Build history of the part. All positions in model axes, mm. Face numbers are marked on the shaded views. A direction names the side the tool comes from. Give positions to 0.01 mm unless a question says otherwise; leave off trailing zeros. Order: outer loops, then holes, each group sorted by start corner. A loop starts at its lowest first (then second) coordinate and runs counter-clockwise, first axis right, second up. Notation, with made-up numbers: (-18.75, 58) - (20.25, 58) arc R18 ccw to (20.25, 71) - close; hole circle Ø5 at (-30, -0.5). An arc over 180 degrees is marked (long way). Answer in a Markdown table with one row per item.
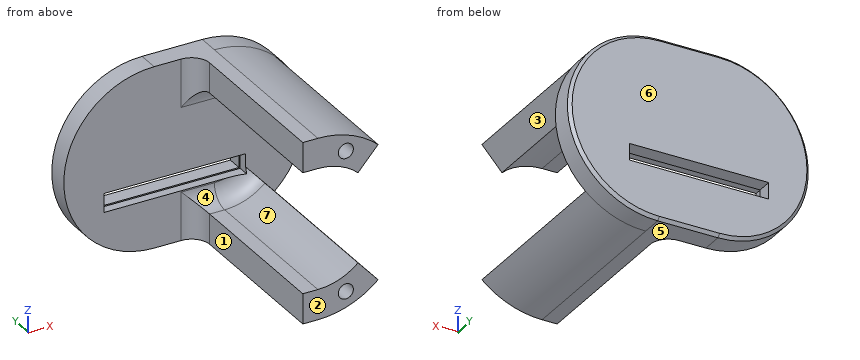
```python
from build123d import *

# Parameters (mm, degrees)
AUFSATZ_LINEAR_AUSTRAGEN1_DEPTH   = 30
AUFSATZ_LINEAR_AUSTRAGEN1_2_DEPTH = 30
AUFSATZ_LINEAR_AUSTRAGEN2_DEPTH   = 4
VERRUNDUNG1_R                     = 3
VERRUNDUNG2_R                     = 3
FASE1_SIZE                        = 0.5
SKIZZE3_R                         = 1.25
SCHNITT_LINEAR_AUSTRAGEN1_DEPTH   = 8
SKIZZE4_W                         = 23.1
SKIZZE4_H                         = 2.74
SCHNITT_LINEAR_AUSTRAGEN2_DEPTH   = 2.5
SCHNITT_LINEAR_AUSTRAGEN3_REACH   = 33.5
SKIZZE5_W                         = 23.5
SKIZZE5_H                         = 3.14


with BuildPart() as part:
    # Skizze1 → Aufsatz-Linear austragen1 (new body)
    with BuildSketch(Plane(origin=(0, 0, 0), x_dir=(1, 0, 0), z_dir=(0, 1, 0))):
        with BuildLine():
            Line((5, 15), (2.5, 15))
            Line((2.5, 15), (2.5, 10))
            Line((2.5, 10), (5, 10))
            ThreePointArc((5, 10), (8.568220898, 9.34172359), (11.666666667, 7.453559925))
            Line((11.666666667, 7.453559925), (15, 11.180339887))
            ThreePointArc((15, 11.180339887), (10.352331347, 14.012585384), (5, 15))
        make_face()
    extrude(amount=-AUFSATZ_LINEAR_AUSTRAGEN1_DEPTH)



with BuildPart() as body_2:
    # Skizze1 → Aufsatz-Linear austragen1 2 (new body)
    with BuildSketch(Plane(origin=(0, 0, 0), x_dir=(1, 0, 0), z_dir=(0, 1, 0))):
        with BuildLine():
            Line((11.666666667, -7.453559925), (15, -11.180339887))
            ThreePointArc((15, -11.180339887), (10.352331347, -14.012585384), (5, -15))
            Line((5, -15), (2.5, -15))
            Line((2.5, -15), (2.5, -10))
            Line((2.5, -10), (5, -10))
            ThreePointArc((5, -10), (8.568220898, -9.34172359), (11.666666667, -7.453559925))
        make_face()
    extrude(amount=-AUFSATZ_LINEAR_AUSTRAGEN1_2_DEPTH)


with BuildPart() as part_1:
    add(part.part)

    add(body_2.part)  # Aufsatz-Linear austragen2 merges body 2
    # Skizze2 → Aufsatz-Linear austragen2 (add)
    with BuildSketch(Plane(origin=(0, 0, 0), x_dir=(1, 0, 0), z_dir=(0, 1, 0))):
        with BuildLine():
            Line((-5, 15), (5, 15))
            ThreePointArc((5, 15), (20, 0), (5, -15))
            Line((5, -15), (-5, -15))
            ThreePointArc((-5, -15), (-20, 0), (-5, 15))
        make_face()
    extrude(amount=AUFSATZ_LINEAR_AUSTRAGEN2_DEPTH)

    # Verrundung1
    verrundung1_edges = [part_1.edges().sort_by_distance(p)[0] for p in [
        (8.568220898, 0, 9.34172359),
        (3.75, 0, 10),
        (8.568220898, 0, -9.34172359),
        (3.75, 0, -10),
    ]]
    fillet(verrundung1_edges, radius=VERRUNDUNG1_R)

    # Verrundung2
    verrundung2_edges = [part_1.edges().sort_by_distance(p)[0] for p in [
        (2.5, 0, 12.5),
        (2.5, 0, -12.5),
    ]]
    fillet(verrundung2_edges, radius=VERRUNDUNG2_R)

    # Fase1
    fase1_edges = [part_1.edges().sort_by_distance(p)[0] for p in [
        (-20, 4, 0),
        (0, 4, 15),
        (20, 4, 0),
        (0, 4, -15),
    ]]
    chamfer(fase1_edges, length=FASE1_SIZE)

    # Skizze3 → Schnitt-Linear austragen1 (cut)
    with BuildSketch(Plane.XZ.offset(30)):
        with Locations((9.644187298, -11.605236936)):
            Circle(SKIZZE3_R)
        with Locations((9.644187298, 11.605236936)):
            Circle(SKIZZE3_R)
    extrude(amount=-SCHNITT_LINEAR_AUSTRAGEN1_DEPTH, mode=Mode.SUBTRACT)

    # Skizze4 → Schnitt-Linear austragen2 (cut)
    with BuildSketch(Plane(origin=(0, 4, 0), x_dir=(1, 0, 0), z_dir=(0, 1, 0))):
        with Locations((-1.602471757, 5.205199937)):
            Rectangle(SKIZZE4_W, SKIZZE4_H)
    extrude(amount=-SCHNITT_LINEAR_AUSTRAGEN2_DEPTH, mode=Mode.SUBTRACT)

    # Skizze5 → Schnitt-Linear austragen3 (cut, up to next)
    with BuildSketch(Plane(origin=(0, 1.5, 0), x_dir=(1, 0, 0), z_dir=(0, 1, 0)), mode=Mode.PRIVATE) as schnitt_linear_austragen3_sk1:
        with Locations((-1.602471757, 5.205199937)):
            Rectangle(SKIZZE5_W, SKIZZE5_H)
    schnitt_linear_austragen3_tool1 = extrude(schnitt_linear_austragen3_sk1.sketch, amount=-SCHNITT_LINEAR_AUSTRAGEN3_REACH, mode=Mode.PRIVATE) & part_1.part
    add(schnitt_linear_austragen3_tool1.solids().sort_by_distance((-1.602472, 1.5, -5.2052))[0], mode=Mode.SUBTRACT)


solid = part_1.part
```
1. Cut at C-C on y = -2.5. Write the cut outline in (x, z).
Check result:
| item | result |
|---|---|
| outline | (2.46, -15) - (5, -15) arc R15 ccw to (15, -11.18) - (11.64, -7.42) arc R9.96 cw to (5, -9.96) - (2.46, -9.96) - close; (2.46, 9.96) - (5, 9.96) arc R9.96 cw to (11.64, 7.42) - (15, 11.18) arc R15 ccw to (5, 15) - (2.46, 15) - close |
2. Which spindle directions (+Z, -Z, +X, -X, +Y, -Y) get a long thin tool onto all of the face, cutting with end or side? Do the marked faces 1, 2, 3 and 4. Say none if no direction does.
Check result:
| item | result |
|---|---|
| face 1 | +Z, -Z, -X, -Y |
| face 2 | +Z, -Z, +X, -X, -Y |
| face 3 | +X, -Y |
| face 4 | -X, -Y |
3. Cut at D-D on x = -2.5. Write the cut outline in (y, z), and give its area (3 significant figures).
Check result:
| item | result |
|---|---|
| outline | (0, -15) - (3.5, -15) - (4, -14.5) - (4, -6.58) - (1.5, -6.58) - (1.5, -6.78) - (0, -6.78) - close; (0, -3.64) - (1.5, -3.64) - (1.5, -3.84) - (4, -3.84) - (4, 14.5) - (3.5, 15) - (0, 15) - close |
| area | 108 mm² |
4. Drop flat-ended pins along their axis: P1, Ø1.5, axis at x = -1.5, y = -2.5, coming from the +Z side; P2, Ø3.5, axis at x = -2.5, z = -4.5, coming from the -Y side; P3, Ø5.5, axis at y = -14.5, z = -13, coming from the -X side; P4, Ø1.2, axis at y = 0.5, z = -5.5, coming from the +X side. Give the stop position or say it passes through.
Check result:
| item | result |
|---|---|
| P1 | passes through |
| P2 | stops at y = 0 |
| P3 | stops at x = 2.5 |
| P4 | stops at x = 19.18 |
5. Cut at A-A on x = 4.5. Write the cut outline in (y, z).
Check result:
| item | result |
|---|---|
| outline | (-30, -15) - (3.5, -15) - (4, -14.5) - (4, -6.58) - (1.5, -6.58) - (1.5, -6.78) - (0, -6.78) - (0, -7) arc R3 cw to (-3, -10) - (-30, -10) - close; (-30, 10) - (-3, 10) arc R3 cw to (0, 7) - (0, -3.64) - (1.5, -3.64) - (1.5, -3.84) - (4, -3.84) - (4, 14.5) - (3.5, 15) - (-30, 15) - close |
6. Two-plate mould, pull along Z, no slides. Class the marked faces 5, 6 and 7: +Z half, -Z half, draft (parallel to the pull), parting line (faces both ways), or undercut.
Check result:
| item | result |
|---|---|
| face 5 | -Z half |
| face 6 | draft |
| face 7 | undercut |
7. Cut at B-B on z = 0. Write the cut outline in (x, y), and give its area (3 significant figures).
Check result:
| item | result |
|---|---|
| outline | (-20, 0) - (20, 0) - (20, 3.5) - (19.5, 4) - (-19.5, 4) - (-20, 3.5) - close |
| area | 160 mm² |
8. Probe line 1 (Z direction, x = 5, y = -6.5); line 2 (Z direction, x = 9, y = -23); line 3 (Y direction, x = 14.5, z = 10). List the from-to ranges inside material, lowest first.
Check result:
| item | result |
|---|---|
| line 1 | z = -15 to -10, 10 to 15 |
| line 2 | z = -14.46 to -12.68, -10.53 to -9.17, 9.17 to 10.53, 12.68 to 14.46 |
| line 3 | y = 0 to 4 |
